from build123d import *

# Parameters (mm, degrees)
BOSS_EXTRU_1_DEPTH           = 10
ESQUISSE2_R                  = 3.1
ENL_V_MAT_EXTRU_1_DEPTH      = 3
COQUE2_T                     = -1
CONG_1_R                     = 3
ENL_V_MAT_EXTRU_2_DEPTH      = 10
ESQUISSE4_R                  = 4.199805961
BOSS_EXTRU_2_DEPTH           = 3
ESQUISSE5_W                  = 3.651716426
ESQUISSE5_H                  = 1.9
ENL_V_MAT_EXTRU_3_DEPTH      = 11
ENL_V_MAT_EXTRU_3_DEPTH_BACK = 11
ENL_V_START                  = -0.3
ENL_V_MAT_EXTRU_4_DEPTH      = 4.2


with BuildPart() as part:
    # Esquisse1 → Boss.-Extru.1 (new body)
    with BuildSketch(Plane.XY):
        Polygon((0, -43.836884112), (30.997358022, -30.997358022), (43.836884112, 0), (30.997358022, 30.997358022), (0, 43.836884112), (-30.997358022, 30.997358022), (-43.836884112, 0), (-30.997358022, -30.997358022), align=None)
    extrude(amount=BOSS_EXTRU_1_DEPTH)

    # Esquisse2 → Enl_v. mat.-Extru.1 (cut)
    with BuildSketch(Plane(origin=(0, 0, 0), x_dir=(-1, 0, 0), z_dir=(0, 0, -1))):
        with Locations((0, 35)):
            Circle(ESQUISSE2_R)
        with Locations((35, 0)):
            Circle(ESQUISSE2_R)
        with Locations((0, -35)):
            Circle(ESQUISSE2_R)
        with Locations((-35, 0)):
            Circle(ESQUISSE2_R)
    extrude(amount=-ENL_V_MAT_EXTRU_1_DEPTH, mode=Mode.SUBTRACT)

    # Coque2
    coque2_openings = [part.faces().sort_by_distance(p)[0] for p in [
        (0, 0, 10),
    ]]
    offset(amount=COQUE2_T, openings=coque2_openings, kind=Kind.INTERSECTION)

    # Cong_1
    cong_1_edges = [part.edges().sort_by_distance(p)[0] for p in [
        (30.997358022, -30.997358022, 5),
        (0, -43.836884112, 5),
        (-30.997358022, -30.997358022, 5),
        (-43.836884112, 0, 5),
        (-30.997358022, 30.997358022, 5),
        (0, 43.836884112, 5),
        (30.997358022, 30.997358022, 5),
        (43.836884112, 0, 5),
    ]]
    fillet(cong_1_edges, radius=CONG_1_R)

    # Esquisse3 → Enl_v. mat.-Extru.2 (cut)
    with BuildSketch(Plane(origin=(-36.493241534, 15.115995578, 0), x_dir=(0, 0, -1), z_dir=(0.923879533, -0.382683432, 0))):
        with BuildLine():
            Line((-7.666279935, -14.17353482), (-6.84853173, -14.17353482))
            ThreePointArc((-6.84853173, -14.17353482), (-6.465848297, -14.097414353), (-6.141424949, -13.880641601))
            Line((-6.141424949, -13.880641601), (-5.504373219, -13.243589871))
            ThreePointArc((-5.504373219, -13.243589871), (-5.287600467, -12.919166523), (-5.21148, -12.53648309))
            Line((-5.21148, -12.53648309), (-5.21148, -7.262190369))
            ThreePointArc((-5.21148, -7.262190369), (-5.287600467, -6.879506937), (-5.504373219, -6.555083588))
            Line((-5.504373219, -6.555083588), (-6.141424949, -5.918031858))
            ThreePointArc((-6.141424949, -5.918031858), (-6.465848297, -5.701259107), (-6.84853173, -5.625138639))
            Line((-6.84853173, -5.625138639), (-7.666279935, -5.625138639))
            ThreePointArc((-7.666279935, -5.625138639), (-8.373386716, -5.918031858), (-8.666279935, -6.625138639))
            Line((-8.666279935, -6.625138639), (-8.666279935, -13.17353482))
            ThreePointArc((-8.666279935, -13.17353482), (-8.373386716, -13.880641601), (-7.666279935, -14.17353482))
        make_face()
    extrude(amount=-ENL_V_MAT_EXTRU_2_DEPTH, mode=Mode.SUBTRACT)

    # Esquisse4 → Boss.-Extru.2 (add)
    with BuildSketch(Plane.XY.offset(1)):
        with Locations((19.756285748, -21.963635985)):
            Circle(ESQUISSE4_R)
    extrude(amount=BOSS_EXTRU_2_DEPTH)

    # Esquisse5 → Enl_v. mat.-Extru.3 (cut, two sides)
    with BuildSketch(Plane(origin=(30.661101875, 30.661101875, 0), x_dir=(-0.707106781, 0.707106781, 0), z_dir=(-0.707106781, -0.707106781, 0))) as enl_v_mat_extru_3_sk:
        with Locations((0.007298531, -7.61148)):
            Rectangle(ESQUISSE5_W, ESQUISSE5_H)
    extrude(amount=ENL_V_MAT_EXTRU_3_DEPTH, mode=Mode.SUBTRACT)
    extrude(enl_v_mat_extru_3_sk.sketch, amount=-ENL_V_MAT_EXTRU_3_DEPTH_BACK, mode=Mode.SUBTRACT)

    # Esquisse6 → Enl_v. mat.-Extru.4 (cut)
    with BuildSketch(Plane.XY.offset(10).offset(ENL_V_START)):
        Polygon((26.258054531, 32.527484923), (32.482135733, 26.303403722), (28.600771667, 22.422039656), (22.376690466, 28.646120858), align=None)
    extrude(amount=-ENL_V_MAT_EXTRU_4_DEPTH, mode=Mode.SUBTRACT)


solid = part.part
Geometry check sheet. Reference: the model listing, model coordinates, mm. A direction names the side the tool comes from. Round coordinates to 2 decimals unless told otherwise and drop trailing zeros. Order: outer loops, then holes, each group sorted by start corner. A loop starts at its lowest first (then second) coordinate and runs counter-clockwise, first axis right, second up. Notation, with made-up numbers: M -23,17.25 L -13,17.25 A25 cw -13,46.25 Z; hole C 80.5,-28.5 d3. An arc over 180 degrees is marked long. Write each question's results on one line, items separated by ' | '. Start each with the question number.
1. Go/stop test with flat-tipped pins: P1, Ø12, axis at x = -5.5, y = -16.5, coming from the +Z side; P2, Ø2.5, axis at x = 30.5, y = 29.5, coming from the +Z side; P3, Ø1.5, axis at x = 34.5, z = 8.5, coming from the +Y side; P4, Ø5.5, axis at x = 0, y = -35, coming from the -Z side. Record where each tip stops, or that it passes through.
2. Cross-section at A-A on x = 35. Record the boundary of the cut face in (y, z), plus the area to 3 significant figures.
3. Cross-section at C-C on x = -28. Record the boundary of the cut face in (y, z), plus the area to 3 significant figures.
4. Draft check along Y on faces 1 (the face through (14.904, -36.581, 5.437)), 2 (the face through (-39, 10, 10)), 3 (the face through (35, 0, 4)), 4 (the face through (-15.7, -37.334, 4.93)). Enter one of: pulls with the +Y half, pulls with the -Y half, needs draft (parallel to the pull), parting line crosses it, or undercut.
5. Cross-section at D-D on x = 11. Record the boundary of the cut face in (y, z).
6. Material ranges on L1, parallel to Y at x = 0, z = 0.7; L2, parallel to Z at x = 28.5, y = 13.5; L3, parallel to Y at x = 29.5, z = 5.5, recorded low to high. Write a range as from..to.
7. Set-up check for faces 5 (the face through (0.404, 38.074, 1.479)), 6 (the face through (3.022, 37.771, 2.479)), 7 (the face through (0.02, 43.59, 5.07)): record each of +Z, -Z, +X, -X, +Y, -Y from which the full face is reachable in a straight line by a thin tool's end or side.
Resolved:
1) P1: z = 1 | P2: z = 10 | P3: y = 24.35 | P4: z = 3
2) outline: M -21.33,0 L -3.1,0 L -3.1,3 L 3.1,3 L 3.1,0 L 21.33,0 L 21.33,10 L 18.72,10 L 18.72,1 L 4.1,1 L 4.1,4 L -4.1,4 L -4.1,1 L -18.72,1 L -18.72,10 L -21.33,10 Z | area: 95.7 mm2
3) outline: M -32.24,0 L 32.24,0 L 32.24,10 L 31.16,10 L 31.16,1 L -31.16,1 L -31.16,10 L -32.24,10 Z | area: 84.0 mm2
4) face 1: undercut | face 2: needs draft | face 3: undercut | face 4: pulls with the -Y half
5) outline: M -39.28,0 L 39.28,0 L 39.28,10 L 38.2,10 L 38.2,1 L -38.2,1 L -38.2,10 L -39.28,10 Z
6) L1: -43.59..-38.1, -31.9..31.9, 38.1..43.59 | L2: 0..1 | L3: -31.62..-30.54, 30.54..31.62
7) face 5: -Z | face 6: +Z | face 7: +Z, -Z, +Y
